Design review of the part built by this model. Coordinates are the model's own, in mm. Face numbers are marked on the shaded views. A direction names the side the tool comes from. Give positions to 0.01 mm unless a question says otherwise; leave off trailing zeros. Loops run counter-clockwise (first coordinate to the right, second up) from the corner with the lowest first, then second, coordinate; pieces in that order, holes last. Notation, with made-up numbers: (32, 17) -> (73, 17) arc R19 cw to (73, 42) -> close; hole circle Ø11 at (-13, 72). An arc over 180 degrees is marked (long way). Answer in a Markdown table with one row per item. Add a question column.
(1) For pin 1 (6 mm diameter, centred on x = -7, z = -26, fed in from +Y); pin 2 (2 mm diameter, centred on x = -42.5, z = -12, fed in from +Y); pin 3 (5 mm diameter, centred on x = -2, z = -5, fed in from -Y), all flat-tipped, find the tip position at first contact; note any pin that passes through.
(2) For the marked faces 1, 2 and 3, list the 3-axis set-ups (+Z, -Z, +X, -X, +Y, -Y) from which the entire face can be reached by the end or side of a thin tool; tool diameter is ignored.
(3) Draft analysis for pull direction Y (two halves, no side actions). For the marked faces 4, 5 and 6, state which applies: +Y half, -Y half, draft (parallel to the pull), parting line (faces both ways), or undercut.
(4) Consider section B-B on z = 10. Write out the cut boundary in (x, y).
(5) Consider section A-A on y = -17.5. Write out the cut boundary in (x, z).
(6) For line 1 (X direction, y = 1.5, z = 15); line 2 (X direction, y = -23, z = -28), list the stretches that pass through material, from the lowest coordinate up.
(7) Consider section C-C on x = -13. Count the separate pieces of the cut face and the enclosed holes in it, then the cut area to 3 significant figures.
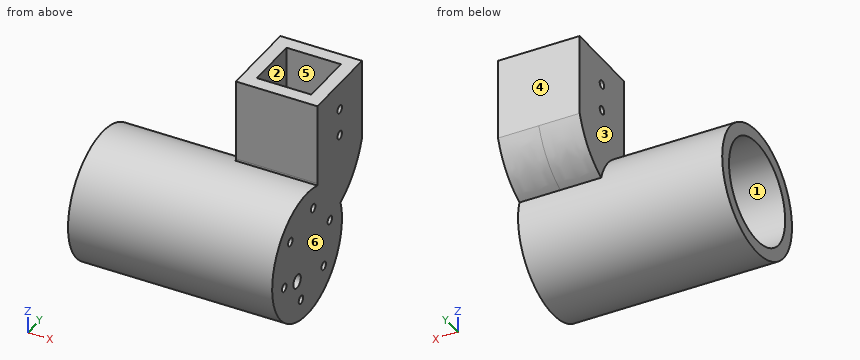
from build123d import *

# Parameters (mm, degrees)
SKETCH1_W           = 30
SKETCH1_H           = 30
SKETCH1_W_2         = 20
SKETCH1_H_2         = 20
BOSS_EXTRUDE1_DEPTH = 30
SKETCH21_R          = 1.5
CUT_EXTRUDE1_DEPTH  = 46
SKETCH22_W          = 30
SKETCH22_H          = 30
BOSS_EXTRUDE2_DEPTH = 5
BOSS_EXTRUDE4_DEPTH = 15
SKETCH26_R          = 23.5
BOSS_EXTRUDE5_DEPTH = 75
SKETCH27_R          = 18.9
CUT_EXTRUDE2_DEPTH  = 100.378046072
SKETCH28_R          = 18.9
BOSS_EXTRUDE6_DEPTH = 5
SKETCH29_R          = 1.5
SKETCH29_R_2        = 2.5
CUT_EXTRUDE3_DEPTH  = 8


with BuildPart() as part:
    # Sketch1 → Boss-Extrude1 (new body)
    with BuildSketch(Plane.XY):
        Rectangle(SKETCH1_W, SKETCH1_H)
        Rectangle(SKETCH1_W_2, SKETCH1_H_2, mode=Mode.SUBTRACT)
    extrude(amount=BOSS_EXTRUDE1_DEPTH)

    # Sketch21 → Cut-Extrude1 (cut, through all)
    with BuildSketch(Plane(origin=(15, 0, 0), x_dir=(0, 0, -1), z_dir=(1, 0, 0))):
        with Locations(Location((-10, 0, 0), (0, 0, 90))):
            Circle(SKETCH21_R)
        with Locations(Location((-20, 0, 0), (0, 0, 90))):
            Circle(SKETCH21_R)
    extrude(amount=-CUT_EXTRUDE1_DEPTH, mode=Mode.SUBTRACT)

    # Sketch22 → Boss-Extrude2 (add)
    with BuildSketch(Plane(origin=(0, 0, 0), x_dir=(-1, 0, 0), z_dir=(0, 0, -1))):
        Rectangle(SKETCH22_W, SKETCH22_H)
    extrude(amount=-BOSS_EXTRUDE2_DEPTH)

    # Sketch25 → Boss-Extrude4 (add, symmetric)
    with BuildSketch(Plane(origin=(0, 0, 0), x_dir=(0, 0, -1), z_dir=(1, 0, 0))):
        with BuildLine():
            Line((0, 15), (0, -15))
            ThreePointArc((0, -15), (1.913417162, -15.380602337), (3.535533906, -16.464466094))
            Line((3.535533906, -16.464466094), (22.852181054, -35.781113242))
            Line((22.852181054, -35.781113242), (36.994316678, -21.638977618))
            Line((36.994316678, -21.638977618), (17.67766953, -2.32233047))
            add(Edge.make_bspline(
                [(0, 15), (13.071207338, 10.453425887), (17.67766953, -2.32233047)],
                knots=[0, 0, 0, 1, 1, 1], degree=2))
        make_face()
    extrude(amount=BOSS_EXTRUDE4_DEPTH, both=True)

    # Sketch26 → Boss-Extrude5 (add)
    with BuildSketch(Plane(origin=(15, 0, 0), x_dir=(0, 0, -1), z_dir=(1, 0, 0))):
        with Locations(Location((23.205734445, -21.992531009, 0), (0, 0, 90))):
            Circle(SKETCH26_R)
    extrude(amount=-BOSS_EXTRUDE5_DEPTH)

    # Sketch27 → Cut-Extrude2 (cut, through all)
    with BuildSketch(Plane(origin=(15, 0, 0), x_dir=(0, 0, -1), z_dir=(1, 0, 0))):
        with Locations(Location((23.205734445, -21.992531009, 0), (0, 0, 90))):
            Circle(SKETCH27_R)
    extrude(amount=-CUT_EXTRUDE2_DEPTH, mode=Mode.SUBTRACT)

    # Sketch28 → Boss-Extrude6 (add)
    with BuildSketch(Plane(origin=(15, 0, 0), x_dir=(0, 0, -1), z_dir=(1, 0, 0))):
        with Locations(Location((23.205734445, -21.992531009, 0), (0, 0, 90))):
            Circle(SKETCH28_R)
    extrude(amount=-BOSS_EXTRUDE6_DEPTH)

    # Sketch29 → Cut-Extrude3 (cut)
    with BuildSketch(Plane(origin=(15, 0, 0), x_dir=(0, 0, -1), z_dir=(1, 0, 0))):
        with Locations(Location((34.448732265, -10.749533188, 0), (0, 0, 90))):
            Circle(SKETCH29_R)
        with Locations(Location((38.563955083, -26.107753826, 0), (0, 0, 90))):
            Circle(SKETCH29_R)
        with Locations(Location((27.320957262, -37.350751647, 0), (0, 0, 90))):
            Circle(SKETCH29_R)
        with Locations(Location((11.962736624, -33.23552883, 0), (0, 0, 90))):
            Circle(SKETCH29_R)
        with Locations(Location((7.847513807, -17.877308192, 0), (0, 0, 90))):
            Circle(SKETCH29_R)
        with Locations(Location((19.090511627, -6.634310371, 0), (0, 0, 90))):
            Circle(SKETCH29_R)
        with Locations(Location((29.923248866, -28.71004543, 0), (0, 0, 90))):
            Circle(SKETCH29_R_2)
    extrude(amount=-CUT_EXTRUDE3_DEPTH, mode=Mode.SUBTRACT)


solid = part.part
Values follow:
| question | item | result |
|---|---|---|
| 1 | pin 1 | y = 1.51 |
| 1 | pin 2 | y = -0.82 |
| 1 | pin 3 | y = -39.47 |
| 2 | face 1 | -X |
| 2 | face 2 | +Z |
| 2 | face 3 | +Z, -X, +Y |
| 3 | face 4 | +Y half |
| 3 | face 5 | undercut |
| 3 | face 6 | draft |
| 4 | outline | (-15, -15) -> (15, -15) -> (15, -1.5) -> (10, -1.5) -> (10, -10) -> (-10, -10) -> (-10, -1.5) -> (-15, -1.5) -> close; (-15, 1.5) -> (-10, 1.5) -> (-10, 10) -> (10, 10) -> (10, 1.5) -> (15, 1.5) -> (15, 15) -> (-15, 15) -> close |
| 5 | outline | (-60, -46.27) -> (15, -46.27) -> (15, -9.3) -> (10, -9.3) -> (10, -41.56) -> (-60, -41.56) -> close; (-60, -4.85) -> (10, -4.85) -> (10, -6.4) -> (15, -6.4) -> (15, -0.14) -> (-60, -0.14) -> close |
| 6 | line 1 | -15 to -10, 10 to 15 |
| 6 | line 2 | 10 to 15 |
| 7 | separate pieces | 1 |
| 7 | enclosed holes | 3 |
| 7 | area | 1,740 mm2 |
